Work out the finished part from the listing and answer in its coordinate system (mm). Face numbers are marked on the shaded views. A direction names the side the tool comes from. Give positions to 0.01 mm unless a question says otherwise; leave off trailing zeros. Order: outer loops, then holes, each group sorted by start corner. A loop starts at its lowest first (then second) coordinate and runs counter-clockwise, first axis right, second up. Notation, with made-up numbers: (41, 43) -> (67, 43) arc R23 ccw to (67, 73) -> close; hole circle Ø8 at (5.5, -23.75). An arc over 180 degrees is marked (long way). Use a Markdown table: item, result. Add a question column.
Autodesk Inventor part; units mm, degrees
ref_plane "YZ Plane" through (0, 0, 0) normal (1, 0, 0) x (0, 1, 0)
ref_plane "XZ Plane" through (0, 0, 0) normal (0, 1, 0) x (-1, 0, 0)
ref_plane "XY Plane" through (0, 0, 0) normal (0, 0, 1) x (1, 0, 0)
sketch "Skizze1" plane through (0, 0, 0) normal (1, 0, 0) x (0, 1, 0)
  line L0 (52.3929, 62.5179) -> (7.3929, 62.5179)
  line L1 (7.3929, 62.5179) -> (7.3929, 17.5179)
  line L2 (7.3929, 17.5179) -> (52.3929, 17.5179)
  line L3 (52.3929, 17.5179) -> (52.3929, 62.5179)
  point P0 (0, 0)
  dimension "d0" = 45
  dimension "d1" = 45
extrude "Extrusion1" add sketch "Skizze1" along normal blind 10
sketch "Skizze2" plane through (0, 7.3929, 62.5179) normal (0, 0, 1) x (1, 0, 0)
  line L0 (0, 0) -> (10, 0)
  line L1 (0, 45) -> (0, 0)
  line L2 (10, 45) -> (10, 0)
  circle A0 centre (5, 22.5) radius 5
  point P0 (0, -7.3929)
  dimension "d4" = 22.5
  dimension "d7" = 10
  dimension "d18" = 5
extrude "Extrusion2" add sketch "Skizze2" along normal blind 45 contours A0
sketch "Skizze3" plane through (0, 7.3929, 17.5179) normal (0, 0, -1) x (-1, 0, 0)
  line L0 (0, 45) -> (-10, 45)
  circle A0 centre (-5, 22.5) radius 5
  line L1 (0, 0) -> (0, 45)
  point P0 (0, -7.3929)
  dimension "d10" = 22.5
  dimension "d11" = 10
  dimension "d19" = 5
extrude "Extrusion3" add sketch "Skizze3" along normal blind 45
sketch "Skizze4" plane through (10, 0, 0) normal (1, 0, 0) x (0, 0, -1)
  point P0 (0, 0)
sketch "Skizze6" plane through (10, 52.3929, 59.5179) normal (1, 0, 0) x (0, 0, -1)
  point P0 (59.5179, -52.3929)
sketch "Skizze7" plane through (10, 52.3929, 59.5179) normal (1, 0, 0) x (0, 0, -1)
  point P0 (59.5179, -52.3929)
sketch "Skizze10" plane through (10, 0, 0) normal (1, 0, 0) x (0, 0, -1)
  line L0 (-62.5179, 29.8929) -> (-62.5179, 7.3929)
  line L1 (-62.5179, 52.3929) -> (-62.5179, 29.8929)
  line L2 (-17.5179, 52.3929) -> (-62.5179, 52.3929)
  line L3 (-17.5179, 29.8929) -> (-17.5179, 52.3929)
  line L4 (-17.5179, 24.8929) -> (27.4821, 24.8929)
  line L5 (-17.5179, 7.3929) -> (-17.5179, 29.8929)
  line L6 (-62.5179, 7.3929) -> (-17.5179, 7.3929)
  line L7 (-62.5179, 7.3929) -> (-52.5179, 7.3929)
  line L8 (-52.5179, 7.3929) -> (-52.5179, 17.3929)
  line L9 (-52.5179, 17.3929) -> (-62.5179, 17.3929)
  line L10 (-62.5179, 17.3929) -> (-62.5179, 7.3929)
  line L11 (-62.5179, 52.3929) -> (-52.5179, 52.3929)
  line L12 (-52.5179, 52.3929) -> (-52.5179, 42.3929)
  line L13 (-52.5179, 42.3929) -> (-62.5179, 42.3929)
  line L14 (-62.5179, 42.3929) -> (-62.5179, 52.3929)
  line L15 (-17.5179, 7.3929) -> (-17.5179, 29.8929)
  line L16 (-17.5179, 7.3929) -> (-27.5179, 7.3929)
  line L17 (-27.5179, 7.3929) -> (-27.5179, 17.3929)
  line L18 (-27.5179, 17.3929) -> (-17.5179, 17.3929)
  line L19 (-17.5179, 17.3929) -> (-17.5179, 7.3929)
  line L20 (-17.5179, 52.3929) -> (-27.5179, 52.3929)
  line L21 (-27.5179, 52.3929) -> (-27.5179, 42.3929)
  line L22 (-27.5179, 42.3929) -> (-17.5179, 42.3929)
  line L23 (-17.5179, 42.3929) -> (-17.5179, 52.3929)
  point P0 (0, 0)
  dimension "d46" = 10
  dimension "d47" = 10
  dimension "d48" = 10
  dimension "d49" = 10
  dimension "d50" = 10
  dimension "d51" = 10
  dimension "d52" = 10
  dimension "d53" = 10
extrude "Extrusion5" add sketch "Skizze10" along normal blind 8 contours L9 L8 L6 L0 | L1 L2 L12 L13 | L17 L18 L5 L6 | L2 L3 L22 L21
sketch "Skizze11" plane through (0, 29.8929, 62.5179) normal (0, 0, 1) x (1, 0, 0)
  line L0 (11.75, 13.85) -> (16.25, 13.85)
  line L1 (16.25, 13.85) -> (16.25, 21.15)
  line L2 (16.25, 21.15) -> (11.75, 21.15)
  line L3 (11.75, 21.15) -> (11.75, 13.85)
  line L4 (11.75, -21.15) -> (16.25, -21.15)
  line L5 (16.25, -21.15) -> (16.25, -13.85)
  line L6 (16.25, -13.85) -> (11.75, -13.85)
  line L7 (11.75, -13.85) -> (11.75, -21.15)
  line L8 (0, -22.5) -> (18, -22.5)
  line L9 (10, 12.5) -> (18, 12.5)
  line L10 (18, 22.5) -> (18, 12.5)
  point P0 (0, -29.8929)
  dimension "d56" = 4.5
  dimension "d57" = 7.3
  dimension "d58" = 4.5
  dimension "d59" = 7.3
  dimension "d60" = 1.35
  dimension "d61" = 1.35
  dimension "d62" = 1.75
extrude "Extrusion6" cut sketch "Skizze11" against normal blind 8
sketch "Skizze12" plane through (10, 7.3929, 27.5179) normal (0, 0, 1) x (1, 0, 0)
  line L0 (1.75, 1.35) -> (6.25, 1.35)
  line L1 (6.25, 1.35) -> (6.25, 8.65)
  line L2 (6.25, 8.65) -> (1.75, 8.65)
  line L3 (1.75, 8.65) -> (1.75, 1.35)
  line L4 (1.75, 36.35) -> (6.25, 36.35)
  line L5 (6.25, 36.35) -> (6.25, 43.65)
  line L6 (6.25, 43.65) -> (1.75, 43.65)
  line L7 (1.75, 43.65) -> (1.75, 36.35)
  line L8 (8, 10) -> (8, 0)
  line L9 (0, 0) -> (8, 0)
  line L10 (0, 35) -> (8, 35)
  point P0 (-10, -7.3929)
  dimension "d65" = 1.75
  dimension "d66" = 1.35
  dimension "d67" = 7.3
  dimension "d68" = 4.5
  dimension "d69" = 7.3
  dimension "d70" = 4.5
  dimension "d71" = 1.35
extrude "Extrusion7" cut sketch "Skizze12" against normal blind 8
sketch "Skizze13" plane through (0, 0, 0) normal (-1, 0, 0) x (0, 0, 1)
  line L0 (62.5179, 52.3929) -> (62.5179, 29.8929)
  line L1 (17.5179, 52.3929) -> (62.5179, 52.3929)
  line L2 (62.5179, 29.8929) -> (62.5179, 7.3929)
  line L3 (62.5179, 7.3929) -> (17.5179, 7.3929)
  line L4 (17.5179, 7.3929) -> (17.5179, 29.8929)
  line L5 (17.5179, 29.8929) -> (17.5179, 52.3929)
  circle A0 centre (57.5179, 47.3929) radius 2
  circle A1 centre (57.5179, 12.3929) radius 2
  circle A2 centre (22.5179, 47.3929) radius 2
  circle A3 centre (22.5179, 12.3929) radius 2
  point P0 (0, 0)
  dimension "d74" = 5
  dimension "d75" = 5
  dimension "d76" = 5
  dimension "d77" = 5
  dimension "d78" = 5
  dimension "d79" = 5
  dimension "d80" = 5
  dimension "d81" = 5
  dimension "d82" = 4
  dimension "d83" = 4
  dimension "d84" = 4
  dimension "d85" = 4
extrude "Extrusion8" cut sketch "Skizze13" against normal blind 12 contours A0 | A1 | A2 | A3
sketch "Skizze14" plane through (0, 0, 0) normal (-1, 0, 0) x (0, 0, 1)
  point P0 (0, 0)
sketch "Skizze15" plane through (10, 0, 0) normal (1, 0, 0) x (0, 0, -1)
  point P0 (0, 0)
properties part number "Spiegelhalter2.0"
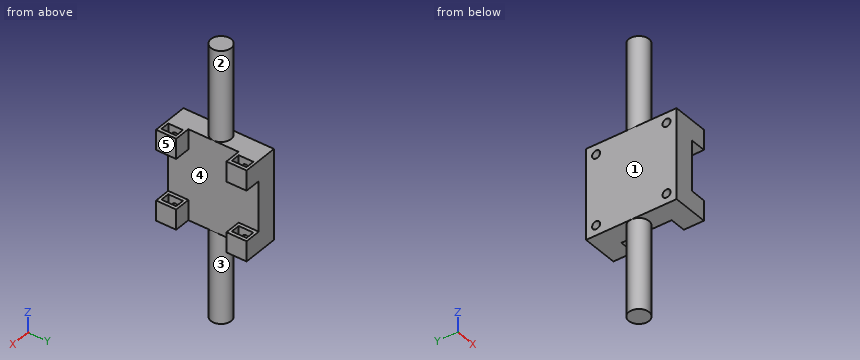
1) The part is cut by section A-A, the plane x = 14.5. State how many separate pieces and enclosed holes the cut face has, then the cut area to 3 significant figures.
2) Which of the six approach directions +Z, -Z, +X, -X, +Y, -Y give full straight-line access (tool end or side, diameter ignored) to the marked faces 1 and 2?
3) Determine the mould class of the marked faces 3, 4 and 5 for opening direction Y: released by +Y, released by -Y, zero draft, split by the parting line, or undercut.
4) The part is cut by section C-C, the plane y = 31.5. Determine the outline of the cut face in (x, z).
5) The part is cut by section D-D, the plane z = 37.5. Determine the outline of the cut face in (x, y).
6) The part is cut by section B-B, the plane x = 3.25. Determine the outline of the cut face in (y, z), then the cut area to 3 significant figures.
7) Flat-ended cylindrical pins translate along their axes: pin 1 (3.5 mm diameter, centred on y = 12.39, z = 57.52, fed in from -X); pin 2 (4 mm diameter, centred on y = 24, z = 78.5, fed in from +X); pin 3 (4 mm diameter, centred on x = 9.5, z = 2.5, fed in from -Y). Find the tip coordinate at first contact, or state that the pin passes through.
8) Straight lines are drawn through the part: line 1 (Y direction, x = 16.75, z = 60.5); line 2 (Z direction, x = 16.75, y = 49); line 3 (Z direction, x = 3, y = 48). For each, find the intervals that lie inside material, in ascending order.
A:
| question | item | result |
|---|---|---|
| 1 | separate pieces | 4 |
| 1 | enclosed holes | 0 |
| 1 | area | 166 mm^2 |
| 2 | face 1 | +Z, -Z, -X, +Y, -Y |
| 2 | face 2 | +Z |
| 3 | face 3 | split by the parting line |
| 3 | face 4 | undercut |
| 3 | face 5 | zero draft |
| 4 | outline | (0, 17.52) -> (0.27, 17.52) -> (0.27, -27.48) -> (9.73, -27.48) -> (9.73, 17.52) -> (10, 17.52) -> (10, 62.52) -> (9.73, 62.52) -> (9.73, 107.52) -> (0.27, 107.52) -> (0.27, 62.52) -> (0, 62.52) -> close |
| 5 | outline | (0, 7.39) -> (10, 7.39) -> (10, 52.39) -> (0, 52.39) -> close |
| 6 | outline | (7.39, 17.52) -> (25.21, 17.52) -> (25.21, -27.48) -> (34.58, -27.48) -> (34.58, 17.52) -> (52.39, 17.52) -> (52.39, 62.52) -> (34.58, 62.52) -> (34.58, 107.52) -> (25.21, 107.52) -> (25.21, 62.52) -> (7.39, 62.52) -> close; hole circle Ø4 at (12.39, 22.52); hole circle Ø4 at (12.39, 57.52); hole circle Ø4 at (47.39, 22.52); hole circle Ø4 at (47.39, 57.52) |
| 6 | area | 2,820 mm^2 |
| 7 | pin 1 | x = 16.25 |
| 7 | pin 2 | x = 8.14 |
| 7 | pin 3 | y = 25.56 |
| 8 | line 1 | 7.39 to 17.39, 42.39 to 52.39 |
| 8 | line 2 | 17.52 to 27.52, 52.52 to 62.52 |
| 8 | line 3 | 17.52 to 20.61, 24.42 to 55.61, 59.42 to 62.52 |
